Autodesk Inventor part; units mm, degrees
ref_plane "Arbeitsebene1" through (0, 0, 0) normal (1, 0, 0) x (0, 1, 0)
ref_plane "Arbeitsebene2" through (65, 0, -40) normal (1, 0, 0) x (0, 0, -1)
ref_plane "XZ Plane" through (0, 0, 0) normal (0, 1, 0) x (-1, 0, 0)
sketch "Skizze1" plane through (0, 0, 0) normal (0, 0, 1) x (1, 0, 0)
  line L0 (10, -10) -> (-10, -10)
  line L1 (-10, -10) -> (-10, 10)
  line L2 (-10, 10) -> (10, 10)
  line L3 (10, 10) -> (10, -10)
  line L4 (10, -10) -> (-10, 10) construction
  line L5 (-10, -10) -> (10, 10) construction
  point P0 (0, 0)
  dimension "d0" = 20
  dimension "d1" = 20
extrude "Extrusion1" add sketch "Skizze1" along normal blind 400
ref_plane "Arbeitsebene1" through (0, 0, 0) normal (1, 0, 0) x (0, 1, 0)
sketch "Skizze2" plane through (0, 0, 0) normal (1, 0, 0) x (0, 1, 0)
  line L0 (10, 0) -> (-10, 0)
  line L1 (10, 0) -> (10, 400)
  line L2 (-10, 400) -> (10, 400)
  line L3 (-10, 0) -> (-10, 400)
  circle A0 centre (0, 410) radius 10
  line L4 (-10, 400) -> (10, 400)
  point P0 (0, 0)
  point P1 (0, 400)
  dimension "d5" = 20
extrude "Extrusion2" add sketch "Skizze2" along normal mid plane 350 contours A0
sketch "Skizze4" plane through (10, 10, 400) normal (1, 0, 0) x (0, 0, -1)
  circle A0 centre (-10, -10) radius 10
  line L0 (400, 0) -> (400, -20)
  line L1 (400, 0) -> (0, 0)
  line L2 (0, -10) -> (0, 0)
  line L3 (0, -20) -> (0, -10)
  line L4 (400, -20) -> (0, -20)
  line L5 (0, -20) -> (0, -10)
  line L6 (0, -12.0268) -> (-0.2075, -12.0268)
  arc A1 (0, -20) -> (-3.0565, -17.1964) centre (-6.4849, -24.002) ccw
  circle A2 centre (-10, -10) radius 10
  arc A3 (-3.0565, -17.1964) -> (-0.2075, -12.0268) centre (-10, -10) ccw
  line L7 (0, -20) -> (0, -12.0268)
  point P0 (400, -10)
extrude "Extrusion3" add sketch "Skizze4" against normal blind 20 contours A0 L6 L3 A1
mirror "Spiegeln1" about plane through (0, 0, 0) normal (0, 1, 0) of "Extrusion3"
fillet "Rundung1" radius 1 4 edges at (10, -10, 200) (-10, -10, 200) (-10, 10, 200) (10, 10, 200)
fillet "Rundung2" radius 3 2 edges at (175, -10, 410) (-175, -10, 410)
sketch "Skizze5" plane through (0, 0, 0) normal (0, 0, -1) x (-1, 0, 0)
  line L0 (-100, -15) -> (100, -15)
  line L1 (100, -15) -> (100, 15)
  line L2 (100, 15) -> (-100, 15)
  line L3 (-100, 15) -> (-100, -15)
  line L4 (-100, -15) -> (100, 15) construction
  line L5 (100, -15) -> (-100, 15) construction
  point P0 (0, 0)
  dimension "d12" = 30
  dimension "d13" = 200
extrude "Extrusion4" add sketch "Skizze5" along normal blind 10
sketch "Skizze6" plane through (0, 0, 0) normal (0, 0, 1) x (1, 0, 0)
  line L0 (100, -15) -> (-100, -15)
  line L1 (100, 15) -> (100, -15)
  line L2 (-100, 15) -> (100, 15)
  line L3 (-100, -15) -> (-100, 15)
  arc A0 (-10, -9) -> (-9, -10) centre (-9, -9) ccw
  line L4 (-10, -9) -> (-10, 9)
  arc A1 (-9, 10) -> (-10, 9) centre (-9, 9) ccw
  line L5 (-9, 10) -> (9, 10)
  arc A2 (10, 9) -> (9, 10) centre (9, 9) ccw
  line L6 (10, 9) -> (10, -9)
  arc A3 (9, -10) -> (10, -9) centre (9, -9) ccw
  line L7 (9, -10) -> (-9, -10)
  circle A4 centre (65, 0) radius 5
  circle A5 centre (-65, 0) radius 5
  line L8 (10, 9) -> (10, -9)
  point P0 (0, 0)
  point P1 (10, 0)
  point P2 (-10, 0)
  dimension "d16" = 130
  dimension "d17" = 65
  dimension "d18" = 10
  dimension "d19" = 10
extrude "Extrusion5" add sketch "Skizze6" along normal blind 10 contours A4 | A5
sketch "Skizze7" plane through (0, 0, -10) normal (0, 0, -1) x (-1, 0, 0)
  circle A0 centre (-65, 0) radius 5
  circle A1 centre (65, 0) radius 5
  point P0 (0, 0)
extrude "Extrusion6" add sketch "Skizze7" along normal blind 30
chamfer "Fase1" distance 4 angle 45 4 edges at (70, 0, -10) (60, 0, 0) (-70, 0, 0) (-60, 0, -10)
sketch "Skizze8" plane through (65, 0, -40) normal (0, 0, -1) x (-1, 0, 0)
  circle A0 centre (0, 0) radius 5
  circle A1 centre (0, 0) radius 5
  point P0 (65, 0)
ref_plane "Arbeitsebene2" through (65, 0, -40) normal (1, 0, 0) x (0, 0, -1)
sketch "Skizze9" plane through (65, 0, -40) normal (1, 0, 0) x (0, 0, -1)
  line L0 (-30, 15) -> (-30, -15)
  line L1 (0, -5) -> (0, 5)
  line L2 (0, 0) -> (10, 0)
  line L3 (30, 20) -> (30, 30)
  arc A0 (10, 0) -> (30, 20) centre (10, 20) ccw
  point P0 (-40, 0)
  point P1 (-30, 0)
  point P2 (30, 0)
  dimension "d29" = 30
  dimension "d30" = 30
  dimension "d31" = 20
sweep "Sweeping1" add profiles "Skizze8" path "Skizze9" path curves L2 A0 L3
mirror "Spiegeln2" about plane through (0, 0, 0) normal (1, 0, 0) of "Sweeping1"
properties part number "Schlüssel" material "Stahl, galvanisiert"
Design review of the part built by this model. Coordinates are the model's own, in mm. A direction names the side the tool comes from. Round coordinates to 2 decimals unless told otherwise and drop trailing zeros. Loops run counter-clockwise (first coordinate to the right, second up) from the corner with the lowest first, then second, coordinate; pieces in that order, holes last. Notation, with made-up numbers: (8.25, 1.25) - (47.25, 1.25) arc R31 cw to (47.25, 31.25) - close; hole circle Ø3 at (86.25, 37.25). An arc over 180 degrees is marked (long way). One line per item, written item: value. Start each with the question number.
1) Consider section A-A on x = 65. Give the boundary of the cut face in (y, z).
2) For faces 5 (the cylindrical face through (70, 25, -70)), 6 (the flat face through (1, -15, -5)), 7 (the cylindrical face through (69.619, 1.915, 6.958)), 8 (the flat face through (-100, 0, -5)), 9 (the flat face through (100, 0, -5)), list the 3-axis set-ups (+Z, -Z, +X, -X, +Y, -Y) from which the entire face can be reached by the end or side of a thin tool; tool diameter is ignored.
3) Insertion check: pin 1 Ø14.5 at (x, z) = (-3.5, 102) entering from -Y; pin 2 Ø6 at (y, z) = (14, 250) entering from +X; pin 3 Ø1 at (y, z) = (-5, 101.5) entering from +X; pin 4 Ø8 at (x, z) = (-46, -7) entering from +Y. Each pin has a flat end and moves straight along its axis. Give the tip position at first contact, or say it passes through.
4) Draft analysis for pull direction X (two halves, no side actions). For faces 1 (the cylindrical face through (-70, 0, 7)), 2 (the conical face through (60.15, 2.01, -13.75)), 3 (the flat face through (175, 0, 410)), 4 (the flat face through (-65, 0, 10)), state which applies: +X half, -X half, draft (parallel to the pull), parting line (faces both ways), or undercut.
5) Consider section B-B on z = 410. Give the boundary of the cut face in (x, y), then the cut area to 3 significant figures.
6) To check wall thickness, follow L1, parallel to X at y = -5, z = 337; L2, parallel to Z at x = 84.5, y = -11.5; L3, parallel to Z at x = 160, y = 1. State the ranges of each line that lie inside material, in increasing order. Write a range as from..to.
7) Consider section D-D on z = 256. Give the boundary of the cut face in (x, y), then the cut area to 3 significant figures.
Reported:
1. outline: (-15, -10) - (-9, -10) - (-5, -14) - (-5, -50) arc R25 ccw to (20, -75) - (30, -75) - (30, -65) - (20, -65) arc R15 cw to (5, -50) - (5, -14) - (9, -10) - (15, -10) - (15, 0) - (9, 0) - (5, 4) - (5, 10) - (-5, 10) - (-5, 4) - (-9, 0) - (-15, 0) - close; circle Ø20 at (0, 410)
2. face 5: +Y
2. face 6: +Z, -Z, +X, -X, -Y
2. face 7: none
2. face 8: -Z, -X, +Y, -Y
2. face 9: -Z, +X, +Y, -Y
3. pin 1: stops at y = -10
3. pin 2: passes through
3. pin 3: stops at x = 10
3. pin 4: stops at y = 15
4. face 1: undercut
4. face 2: undercut
4. face 3: +X half
4. face 4: draft
5. outline: (-175, -7) arc R3 ccw to (-172, -10) - (172, -10) arc R3 ccw to (175, -7) - (175, 7) arc R3 ccw to (172, 10) - (-172, 10) arc R3 ccw to (-175, 7) - close
5. area: 6,990 mm^2
6. L1: x = -10..10
6. L2: z = -10..0
6. L3: z = 400.05..419.95
7. outline: (-10, -9) arc R1 ccw to (-9, -10) - (9, -10) arc R1 ccw to (10, -9) - (10, 9) arc R1 ccw to (9, 10) - (-9, 10) arc R1 ccw to (-10, 9) - close
7. area: 399 mm^2
